For this review, take the finished solid that the model builds, in its own axes (mm). A direction names the side the tool comes from. Round coordinates to 2 decimals unless told otherwise and drop trailing zeros. Write each loop counter-clockwise with the first axis right and the second up, starting at its lowest first coordinate (ties: lowest second). Pieces come first, ordered by that corner, then holes. Notation, with made-up numbers: (2.25, 62.25) -> (37.25, 62.25) arc R18 ccw to (37.25, 86.25) -> close; hole circle Ø10 at (-30.75, 73.5). An arc over 180 degrees is marked (long way). Answer in a Markdown table with one row per item.
from build123d import *

# Parameters (mm, degrees)
F0_R     = 12.7
F1_DEPTH = 19.05


with BuildPart() as f1:
    # F0 (on Front) → F1 (new body)
    with BuildSketch(Plane.XZ):
        with BuildLine():
            Line((-43.05991, 46.274296), (-74.80991, 46.274296))
            ThreePointArc((-74.80991, 46.274296), (-79.300038, 44.414424), (-81.15991, 39.924296))
            Line((-81.15991, 39.924296), (-81.15991, -10.875704))
            ThreePointArc((-81.15991, -10.875704), (-79.300038, -15.365832), (-74.80991, -17.225704))
            Line((-74.80991, -17.225704), (-43.05991, -17.225704))
            Line((-43.05991, -17.225704), (-43.05991, -42.625704))
            Line((-43.05991, -42.625704), (7.74009, -42.625704))
            Line((7.74009, -42.625704), (7.74009, -17.225704))
            Line((7.74009, -17.225704), (39.49009, -17.225704))
            ThreePointArc((39.49009, -17.225704), (43.980218, -15.365832), (45.84009, -10.875704))
            Line((45.84009, -10.875704), (45.84009, 39.924296))
            ThreePointArc((45.84009, 39.924296), (43.980218, 44.414424), (39.49009, 46.274296))
            Line((39.49009, 46.274296), (7.74009, 46.274296))
            Line((7.74009, 46.274296), (7.74009, 20.111208))
            Line((7.74009, 20.111208), (-43.05991, 20.111208))
            Line((-43.05991, 20.111208), (-43.05991, 46.274296))
        make_face()
        with Locations((-17.65991, -17.225704)):
            Circle(F0_R, mode=Mode.SUBTRACT)
        with Locations((-62.10991, 14.524296)):
            Circle(F0_R, mode=Mode.SUBTRACT)
        with Locations((26.79009, 14.524296)):
            Circle(F0_R, mode=Mode.SUBTRACT)
    extrude(amount=F1_DEPTH)


solid = f1.part
1) Consider section D-D on y = -5. State the section outline as (x, z) points, then the cut area to 3 significant figures.
Solved:
| item | result |
|---|---|
| outline | (-81.16, -10.88) arc R6.35 ccw to (-74.81, -17.23) -> (-43.06, -17.23) -> (-43.06, -42.63) -> (7.74, -42.63) -> (7.74, -17.23) -> (39.49, -17.23) arc R6.35 ccw to (45.84, -10.88) -> (45.84, 39.92) arc R6.35 ccw to (39.49, 46.27) -> (7.74, 46.27) -> (7.74, 20.11) -> (-43.06, 20.11) -> (-43.06, 46.27) -> (-74.81, 46.27) arc R6.35 ccw to (-81.16, 39.92) -> close; hole circle Ø25.4 at (-62.11, 14.52); hole circle Ø25.4 at (-17.66, -17.23); hole circle Ø25.4 at (26.79, 14.52) |
| area | 6,470 mm² |
2) Consider section B-B on x = 38. State the section outline as (y, z) points.
Solved:
| item | result |
|---|---|
| outline | (-19.05, -17.23) -> (0, -17.23) -> (0, 8.56) -> (-19.05, 8.56) -> close; (-19.05, 20.49) -> (0, 20.49) -> (0, 46.27) -> (-19.05, 46.27) -> close |
3) Consider section A-A on z = 29.5. State the section outline as (x, y) points, then the cut area to 3 significant figures.
Solved:
| item | result |
|---|---|
| outline | (-81.16, -19.05) -> (-43.06, -19.05) -> (-43.06, 0) -> (-81.16, 0) -> close; (7.74, -19.05) -> (45.84, -19.05) -> (45.84, 0) -> (7.74, 0) -> close |
| area | 1,450 mm² |
4) For faces 1 (the flat face through (-18, -9, -42.626)), 2 (the flat face through (-59, -9, -17.226)), 3 (the flat face through (7.74, -9, 33)), list the 3-axis set-ups (+Z, -Z, +X, -X, +Y, -Y) from which the entire face can be reached by the end or side of a thin tool; tool diameter is ignored.
Solved:
| item | result |
|---|---|
| face 1 | -Z, +X, -X, +Y, -Y |
| face 2 | -Z, -X, +Y, -Y |
| face 3 | +Z, +Y, -Y |
5) Consider section C-C on z = 4.5. State the section outline as (x, y) points.
Solved:
| item | result |
|---|---|
| outline | (-81.16, -19.05) -> (-69.91, -19.05) -> (-69.91, 0) -> (-81.16, 0) -> close; (-54.31, -19.05) -> (18.99, -19.05) -> (18.99, 0) -> (-54.31, 0) -> close; (34.59, -19.05) -> (45.84, -19.05) -> (45.84, 0) -> (34.59, 0) -> close |
6) Mouldability with a two-part tool opening along Z and no side actions: class faces 4 (the flat face through (23, -9, -17.226)), 5 (the flat face through (-19, 0, 12)), 6 (the cylindrical face through (-30.348, -9.392, -16.667)) as pulls with the +Z half, pulls with the -Z half, needs draft (parallel to the pull), parting line crosses it, or undercut.
Solved:
| item | result |
|---|---|
| face 4 | pulls with the -Z half |
| face 5 | needs draft |
| face 6 | undercut |
7) For line 1 (Z direction, x = -17, y = -11.5); line 2 (X direction, y = -8.5, z = 8.5); line 3 (X direction, y = -1.75, z = 38), list the stretches that pass through material, from the lowest coordinate up. Write a range as [from, to].
Solved:
| item | result |
|---|---|
| line 1 | [-42.63, -29.91], [-4.54, 20.11] |
| line 2 | [-81.16, -73.29], [-50.93, 15.61], [37.97, 45.84] |
| line 3 | [-81.16, -43.06], [7.74, 45.84] |
8) Clearance check with flat-ended pins moving along their axes: pin 1 Ø5.5 at (y, z) = (-5.5, -35.5) entering from -X; pin 2 Ø5 at (x, y) = (30.5, -13.5) entering from -Z; pin 3 Ø5.5 at (x, y) = (-8, -11.5) entering from +Z. State where each tip first meets the part, or that it passes through.
Solved:
| item | result |
|---|---|
| pin 1 | x = -43.06 |
| pin 2 | z = -17.23 |
| pin 3 | z = 20.11 |
